Geometry: final body of the model. Coordinates: model frame, mm. Face numbers are marked on the shaded views. A direction names the side the tool comes from. Give positions to 0.01 mm unless a question says otherwise; leave off trailing zeros. Order: outer loops, then holes, each group sorted by start corner. A loop starts at its lowest first (then second) coordinate and runs counter-clockwise, first axis right, second up. Notation, with made-up numbers: M -13,69 L 26,69 A33 cw 26,103 Z; hole C 10.25,-7.5 d10. An arc over 180 degrees is marked long. One line per item, written item: value. Start each with the question number.
```python
from build123d import *

# Parameters (mm, degrees)
SKETCH1_W           = 81.28
SKETCH1_H           = 53.34
BOSS_EXTRUDE1_DEPTH = 22.098
SKETCH2_W           = 27.94
SKETCH2_H           = 22.098
CUT_EXTRUDE1_DEPTH  = 29.591
SKETCH3_W           = 27.94
SKETCH3_H           = 22.098
CUT_EXTRUDE2_DEPTH  = 1.651
SKETCH4_W           = 27.94
SKETCH4_H           = 22.098
CUT_EXTRUDE3_DEPTH  = 29.591
SKETCH5_W           = 27.94
SKETCH5_H           = 22.098
CUT_EXTRUDE4_DEPTH  = 1.651
SKETCH6_W           = 27.94
SKETCH6_H           = 22.098
CUT_EXTRUDE5_DEPTH  = 1.651
CUT_EXTRUDE6_DEPTH  = 8.89
SKETCH8_W           = 27.94
SKETCH8_H           = 22.098
CUT_EXTRUDE7_DEPTH  = 1.651
CUT_EXTRUDE8_DEPTH  = 8.89
SKETCH10_W          = 25.4
SKETCH10_H          = 25.4
BOSS_EXTRUDE2_DEPTH = 1.651
SKETCH11_W          = 25.4
SKETCH11_H          = 25.4
BOSS_EXTRUDE3_DEPTH = 1.651
CUT_EXTRUDE9_DEPTH  = 8.89
CUT_EXTRUDE10_DEPTH = 8.89
CUT_EXTRUDE11_DEPTH = 8.89
CUT_EXTRUDE12_DEPTH = 8.89
CUT_EXTRUDE13_DEPTH = 8.89
CUT_EXTRUDE14_DEPTH = 8.89
CUT_EXTRUDE15_DEPTH = 8.89
CUT_EXTRUDE16_DEPTH = 8.89
CUT_EXTRUDE17_DEPTH = 8.89
CUT_EXTRUDE18_DEPTH = 8.89
SKETCH22_W          = 22.098
SKETCH22_H          = 22.098
BOSS_EXTRUDE4_DEPTH = 27.94
SKETCH23_W          = 15.748
SKETCH23_H          = 15.748
CUT_EXTRUDE19_DEPTH = 27.94
FILLET1_R           = 1.27


with BuildPart() as part:
    # Sketch1 → Boss-Extrude1 (new body)
    with BuildSketch(Plane.XZ.offset(11.049)):
        with Locations((0, 13.97)):
            Rectangle(SKETCH1_W, SKETCH1_H)
    extrude(amount=-BOSS_EXTRUDE1_DEPTH)

    # Sketch2 → Cut-Extrude1 (cut)
    with BuildSketch(Plane.XY.offset(40.64)):
        with Locations((-26.67, 0)):
            Rectangle(SKETCH2_W, SKETCH2_H)
    extrude(amount=-CUT_EXTRUDE1_DEPTH, mode=Mode.SUBTRACT)

    # Sketch3 → Cut-Extrude2 (cut)
    with BuildSketch(Plane(origin=(0, 0, -12.7), x_dir=(-1, 0, 0), z_dir=(0, 0, -1))):
        with Locations((26.67, 0)):
            Rectangle(SKETCH3_W, SKETCH3_H)
    extrude(amount=-CUT_EXTRUDE2_DEPTH, mode=Mode.SUBTRACT)

    # Sketch4 → Cut-Extrude3 (cut)
    with BuildSketch(Plane(origin=(40.64, 0, 0), x_dir=(0, 0, -1), z_dir=(1, 0, 0))):
        with Locations((-26.67, 0)):
            Rectangle(SKETCH4_W, SKETCH4_H)
    extrude(amount=-CUT_EXTRUDE3_DEPTH, mode=Mode.SUBTRACT)

    # Sketch5 → Cut-Extrude4 (cut)
    with BuildSketch(Plane.ZY.offset(12.7)):
        with Locations((26.67, 0)):
            Rectangle(SKETCH5_W, SKETCH5_H)
    extrude(amount=-CUT_EXTRUDE4_DEPTH, mode=Mode.SUBTRACT)

    # Sketch6 → Cut-Extrude5 (cut)
    with BuildSketch(Plane.XY.offset(12.7)):
        with Locations((26.67, 0)):
            Rectangle(SKETCH6_W, SKETCH6_H)
    extrude(amount=-CUT_EXTRUDE5_DEPTH, mode=Mode.SUBTRACT)

    # Sketch7 → Cut-Extrude6 (cut)
    with BuildSketch(Plane(origin=(0, 11.049, 0), x_dir=(-1, 0, 0), z_dir=(0, 1, 0))):
        with BuildLine():
            Line((-12.7, -7.874), (-12.7, 7.874))
            Line((-12.7, 7.874), (-22.1615, 7.874))
            ThreePointArc((-22.1615, 7.874), (-23.1775, 6.858), (-22.1615, 5.842))
            Line((-22.1615, 5.842), (-21.1455, 5.842))
            Line((-21.1455, 5.842), (-21.1455, -5.842))
            Line((-21.1455, -5.842), (-22.1615, -5.842))
            ThreePointArc((-22.1615, -5.842), (-23.1775, -6.858), (-22.1615, -7.874))
            Line((-22.1615, -7.874), (-12.7, -7.874))
        make_face()
    extrude(amount=-CUT_EXTRUDE6_DEPTH, mode=Mode.SUBTRACT)

    # Sketch8 → Cut-Extrude7 (cut)
    with BuildSketch(Plane(origin=(0, 0, -12.7), x_dir=(-1, 0, 0), z_dir=(0, 0, -1))):
        with Locations((-26.67, 0)):
            Rectangle(SKETCH8_W, SKETCH8_H)
    extrude(amount=-CUT_EXTRUDE7_DEPTH, mode=Mode.SUBTRACT)

    # Sketch9 → Cut-Extrude8 (cut)
    with BuildSketch(Plane(origin=(0, 11.049, 0), x_dir=(-1, 0, 0), z_dir=(0, 1, 0))):
        with BuildLine():
            Line((7.874, 12.7), (7.874, 22.1615))
            ThreePointArc((7.874, 22.1615), (6.858, 23.1775), (5.842, 22.1615))
            Line((5.842, 22.1615), (5.842, 21.1455))
            Line((5.842, 21.1455), (-5.842, 21.1455))
            Line((-5.842, 21.1455), (-5.842, 22.1615))
            ThreePointArc((-5.842, 22.1615), (-6.858, 23.1775), (-7.874, 22.1615))
            Line((-7.874, 22.1615), (-7.874, 12.7))
            Line((-7.874, 12.7), (7.874, 12.7))
        make_face()
    extrude(amount=-CUT_EXTRUDE8_DEPTH, mode=Mode.SUBTRACT)

    # Sketch10 → Boss-Extrude2 (add)
    with BuildSketch(Plane(origin=(0, 11.049, 0), x_dir=(-1, 0, 0), z_dir=(0, 1, 0))):
        Rectangle(SKETCH10_W, SKETCH10_H)
    extrude(amount=BOSS_EXTRUDE2_DEPTH)

    # Sketch11 → Boss-Extrude3 (add)
    with BuildSketch(Plane.XZ.offset(11.049)):
        Rectangle(SKETCH11_W, SKETCH11_H)
    extrude(amount=BOSS_EXTRUDE3_DEPTH)

    # Sketch12 → Cut-Extrude9 (cut)
    with BuildSketch(Plane.XZ.offset(11.049)):
        with BuildLine():
            Line((-7.874, 22.1615), (-7.874, 12.7))
            Line((-7.874, 12.7), (7.874, 12.7))
            Line((7.874, 12.7), (7.874, 22.1615))
            ThreePointArc((7.874, 22.1615), (6.858, 23.1775), (5.842, 22.1615))
            Line((5.842, 22.1615), (5.842, 21.1455))
            Line((5.842, 21.1455), (-5.842, 21.1455))
            Line((-5.842, 21.1455), (-5.842, 22.1615))
            ThreePointArc((-5.842, 22.1615), (-6.858, 23.1775), (-7.874, 22.1615))
        make_face()
    extrude(amount=-CUT_EXTRUDE9_DEPTH, mode=Mode.SUBTRACT)

    # Sketch13 → Cut-Extrude10 (cut)
    with BuildSketch(Plane.XZ.offset(11.049)):
        with BuildLine():
            Line((12.7, 7.874), (12.7, -7.874))
            Line((12.7, -7.874), (22.1615, -7.874))
            ThreePointArc((22.1615, -7.874), (23.1775, -6.858), (22.1615, -5.842))
            Line((22.1615, -5.842), (21.1455, -5.842))
            Line((21.1455, -5.842), (21.1455, 5.842))
            Line((21.1455, 5.842), (22.1615, 5.842))
            ThreePointArc((22.1615, 5.842), (23.1775, 6.858), (22.1615, 7.874))
            Line((22.1615, 7.874), (12.7, 7.874))
        make_face()
    extrude(amount=-CUT_EXTRUDE10_DEPTH, mode=Mode.SUBTRACT)

    # Sketch14 → Cut-Extrude11 (cut)
    with BuildSketch(Plane.XZ.offset(11.049)):
        with BuildLine():
            Line((-22.1615, 5.842), (-21.1455, 5.842))
            Line((-21.1455, 5.842), (-21.1455, -5.842))
            Line((-21.1455, -5.842), (-22.1615, -5.842))
            ThreePointArc((-22.1615, -5.842), (-23.1775, -6.858), (-22.1615, -7.874))
            Line((-22.1615, -7.874), (-12.7, -7.874))
            Line((-12.7, -7.874), (-12.7, 7.874))
            Line((-12.7, 7.874), (-22.1615, 7.874))
            ThreePointArc((-22.1615, 7.874), (-23.1775, 6.858), (-22.1615, 5.842))
        make_face()
    extrude(amount=-CUT_EXTRUDE11_DEPTH, mode=Mode.SUBTRACT)

    # Sketch15 → Cut-Extrude12 (cut)
    with BuildSketch(Plane(origin=(0, 11.049, 0), x_dir=(-1, 0, 0), z_dir=(0, 1, 0))):
        with BuildLine():
            Line((21.1455, 5.842), (22.1615, 5.842))
            ThreePointArc((22.1615, 5.842), (23.1775, 6.858), (22.1615, 7.874))
            Line((22.1615, 7.874), (12.7, 7.874))
            Line((12.7, 7.874), (12.7, -7.874))
            Line((12.7, -7.874), (22.1615, -7.874))
            ThreePointArc((22.1615, -7.874), (23.1775, -6.858), (22.1615, -5.842))
            Line((22.1615, -5.842), (21.1455, -5.842))
            Line((21.1455, -5.842), (21.1455, 5.842))
        make_face()
    extrude(amount=-CUT_EXTRUDE12_DEPTH, mode=Mode.SUBTRACT)

    # Sketch16 → Cut-Extrude13 (cut)
    with BuildSketch(Plane.XZ.offset(11.049)):
        with BuildLine():
            Line((-37.465, 7.874), (-37.465, -7.874))
            Line((-37.465, -7.874), (-28.0035, -7.874))
            ThreePointArc((-28.0035, -7.874), (-26.9875, -6.858), (-28.0035, -5.842))
            Line((-28.0035, -5.842), (-29.0195, -5.842))
            Line((-29.0195, -5.842), (-29.0195, 5.842))
            Line((-29.0195, 5.842), (-28.0035, 5.842))
            ThreePointArc((-28.0035, 5.842), (-26.9875, 6.858), (-28.0035, 7.874))
            Line((-28.0035, 7.874), (-37.465, 7.874))
        make_face()
    extrude(amount=-CUT_EXTRUDE13_DEPTH, mode=Mode.SUBTRACT)

    # Sketch17 → Cut-Extrude14 (cut)
    with BuildSketch(Plane.XZ.offset(11.049)):
        with BuildLine():
            Line((28.0035, 5.842), (29.0195, 5.842))
            Line((29.0195, 5.842), (29.0195, -5.842))
            Line((29.0195, -5.842), (28.0035, -5.842))
            ThreePointArc((28.0035, -5.842), (26.9875, -6.858), (28.0035, -7.874))
            Line((28.0035, -7.874), (37.465, -7.874))
            Line((37.465, -7.874), (37.465, 7.874))
            Line((37.465, 7.874), (28.0035, 7.874))
            ThreePointArc((28.0035, 7.874), (26.9875, 6.858), (28.0035, 5.842))
        make_face()
    extrude(amount=-CUT_EXTRUDE14_DEPTH, mode=Mode.SUBTRACT)

    # Sketch18 → Cut-Extrude15 (cut)
    with BuildSketch(Plane(origin=(0, 11.049, 0), x_dir=(-1, 0, 0), z_dir=(0, 1, 0))):
        with BuildLine():
            Line((-29.0195, -5.842), (-29.0195, 5.842))
            Line((-29.0195, 5.842), (-28.0035, 5.842))
            ThreePointArc((-28.0035, 5.842), (-26.9875, 6.858), (-28.0035, 7.874))
            Line((-28.0035, 7.874), (-37.465, 7.874))
            Line((-37.465, 7.874), (-37.465, -7.874))
            Line((-37.465, -7.874), (-28.0035, -7.874))
            ThreePointArc((-28.0035, -7.874), (-26.9875, -6.858), (-28.0035, -5.842))
            Line((-28.0035, -5.842), (-29.0195, -5.842))
        make_face()
    extrude(amount=-CUT_EXTRUDE15_DEPTH, mode=Mode.SUBTRACT)

    # Sketch19 → Cut-Extrude16 (cut)
    with BuildSketch(Plane.XZ.offset(11.049)):
        with BuildLine():
            Line((-7.874, 37.465), (-7.874, 28.0035))
            ThreePointArc((-7.874, 28.0035), (-6.858, 26.9875), (-5.842, 28.0035))
            Line((-5.842, 28.0035), (-5.842, 29.0195))
            Line((-5.842, 29.0195), (5.842, 29.0195))
            Line((5.842, 29.0195), (5.842, 28.0035))
            ThreePointArc((5.842, 28.0035), (6.858, 26.9875), (7.874, 28.0035))
            Line((7.874, 28.0035), (7.874, 37.465))
            Line((7.874, 37.465), (-7.874, 37.465))
        make_face()
    extrude(amount=-CUT_EXTRUDE16_DEPTH, mode=Mode.SUBTRACT)

    # Sketch20 → Cut-Extrude17 (cut)
    with BuildSketch(Plane(origin=(0, 11.049, 0), x_dir=(-1, 0, 0), z_dir=(0, 1, 0))):
        with BuildLine():
            Line((5.842, 29.0195), (5.842, 28.0035))
            ThreePointArc((5.842, 28.0035), (6.858, 26.9875), (7.874, 28.0035))
            Line((7.874, 28.0035), (7.874, 37.465))
            Line((7.874, 37.465), (-7.874, 37.465))
            Line((-7.874, 37.465), (-7.874, 28.0035))
            ThreePointArc((-7.874, 28.0035), (-6.858, 26.9875), (-5.842, 28.0035))
            Line((-5.842, 28.0035), (-5.842, 29.0195))
            Line((-5.842, 29.0195), (5.842, 29.0195))
        make_face()
    extrude(amount=-CUT_EXTRUDE17_DEPTH, mode=Mode.SUBTRACT)

    # Sketch21 → Cut-Extrude18 (cut)
    with BuildSketch(Plane(origin=(0, 11.049, 0), x_dir=(-1, 0, 0), z_dir=(0, 1, 0))):
        with BuildLine():
            Line((28.0035, -7.874), (37.465, -7.874))
            Line((37.465, -7.874), (37.465, 7.874))
            Line((37.465, 7.874), (28.0035, 7.874))
            ThreePointArc((28.0035, 7.874), (26.9875, 6.858), (28.0035, 5.842))
            Line((28.0035, 5.842), (29.0195, 5.842))
            Line((29.0195, 5.842), (29.0195, -5.842))
            Line((29.0195, -5.842), (28.0035, -5.842))
            ThreePointArc((28.0035, -5.842), (26.9875, -6.858), (28.0035, -7.874))
        make_face()
    extrude(amount=-CUT_EXTRUDE18_DEPTH, mode=Mode.SUBTRACT)

    # Sketch22 → Boss-Extrude4 (add)
    with BuildSketch(Plane(origin=(0, 12.7, 0), x_dir=(-1, 0, 0), z_dir=(0, 1, 0))):
        Rectangle(SKETCH22_W, SKETCH22_H)
    extrude(amount=BOSS_EXTRUDE4_DEPTH)

    # Sketch23 → Cut-Extrude19 (cut)
    with BuildSketch(Plane(origin=(0, 40.64, 0), x_dir=(-1, 0, 0), z_dir=(0, 1, 0))):
        Rectangle(SKETCH23_W, SKETCH23_H)
    extrude(amount=-CUT_EXTRUDE19_DEPTH, mode=Mode.SUBTRACT)

    # Fillet1
    fillet1_edges = [part.edges().sort_by_distance(p)[0] for p in [
        (26.67, 11.049, -11.049),
        (26.67, -11.049, -11.049),
        (-26.67, 11.049, 11.049),
        (-26.67, -11.049, 11.049),
        (-26.67, -11.049, -11.049),
        (-26.67, 11.049, -11.049),
        (-11.049, 26.67, -11.049),
        (-11.049, 26.67, 11.049),
        (11.049, 26.67, 11.049),
        (11.049, 26.67, -11.049),
        (11.049, -11.049, 26.67),
        (11.049, 11.049, 26.67),
        (-11.049, 11.049, 26.67),
        (-11.049, -11.049, 26.67),
        (26.67, -11.049, 11.049),
        (26.67, 11.049, 11.049),
    ]]
    fillet(fillet1_edges, radius=FILLET1_R)


solid = part.part
```
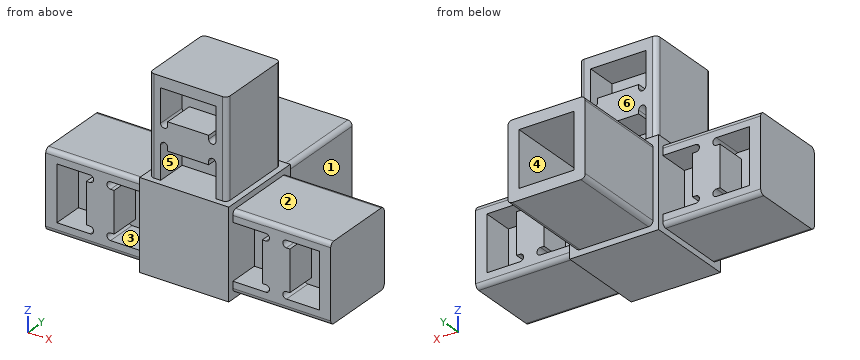
Q1. Set-up query: the marked faces 4, 5 and 6. Return all of +Z, -Z, +X, -X, +Y, -Y with unobstructed straight access to the full face (end or side cutting, diameter ignored); none if empty.
Q2. Mould query, pull axis Z, two halves, no side actions, for the marked faces 1, 2 and 3. Classes: +Z half, -Z half, draft (parallel to the pull), parting line (faces both ways), or undercut.
Q3. Section query D-D on x = 32. Return loops of the section in (y, z), and give its area (3 significant figures).
Q4. Section query C-C on z = 32.5. Return loops of the section in (x, y).
Q5. Ray query, line 1 along X through (y, z) = (9, 2) (1 decimal); line 2 along Z through (x, y) = (-1.5, -9.5) (1 decimal); line 3 along X through (y, z) = (26, -2.5). Return the intervals inside material, ascending. Write a range as [from, to].
Q6. Section query A-A on y = 25.5. Return loops of the section in (x, z), and give its area (3 significant figures).
Q7. Section query B-B on x = 1. Return loops of the section in (y, z) (1 decimal).
Q8. Contact query for flat-ended pins moving along their axis: pin 1 (2 mm diameter, centred on x = -8.5, y = 14.5, fed in from -Z); pin 2 (15.5 mm diameter, centred on y = -3, z = 20.5, fed in from -X); pin 3 (8 mm diameter, centred on x = -1.5, y = 21.5, fed in from +Z). Output: stop coordinate, or through.
Results below:
1. face 4: +Y
1. face 5: -Y
1. face 6: +Z, +X, -X, +Y
2. face 1: draft
2. face 2: +Z half
2. face 3: undercut
3. outline: M -11.05,-9.78 A1.27 ccw -9.78,-11.05 L 9.78,-11.05 A1.27 ccw 11.05,-9.78 L 11.05,-7.87 L 2.16,-7.87 L 2.16,7.87 L 11.05,7.87 L 11.05,9.78 A1.27 ccw 9.78,11.05 L -9.78,11.05 A1.27 ccw -11.05,9.78 L -11.05,7.87 L -2.16,7.87 L -2.16,-7.87 L -11.05,-7.87 Z
3. area: 207 mm2
4. outline: M -11.05,-9.78 A1.27 ccw -9.78,-11.05 L -7.87,-11.05 L -7.87,-2.16 L 7.87,-2.16 L 7.87,-11.05 L 9.78,-11.05 A1.27 ccw 11.05,-9.78 L 11.05,9.78 A1.27 ccw 9.78,11.05 L 7.87,11.05 L 7.87,2.16 L -7.87,2.16 L -7.87,11.05 L -9.78,11.05 A1.27 ccw -11.05,9.78 Z
5. line 1: [-40.6, -37.5], [-29, -21.1], [-12.7, 12.7], [21.1, 29], [37.5, 40.6]
5. line 2: [-12.7, 12.7], [21.1, 29], [37.5, 40.6]
5. line 3: [-11.05, -7.87], [7.87, 11.05]
6. outline: M -11.05,-9.78 A1.27 ccw -9.78,-11.05 L 9.78,-11.05 A1.27 ccw 11.05,-9.78 L 11.05,9.78 A1.27 ccw 9.78,11.05 L -9.78,11.05 A1.27 ccw -11.05,9.78 Z; hole M -7.87,-7.87 L 7.87,-7.87 L 7.87,7.87 L -7.87,7.87 Z
6. area: 239 mm2
7. outline: M -12.7,-12.7 L 12.7,-12.7 L 12.7,-11 L 40.6,-11 L 40.6,-7.9 L 12.7,-7.9 L 12.7,7.9 L 40.6,7.9 L 40.6,11 L 12.7,11 L 12.7,12.7 L 2.2,12.7 L 2.2,21.1 L 11,21.1 L 11,29 L 2.2,29 L 2.2,37.5 L 11,37.5 L 11,40.6 L -11,40.6 L -11,37.5 L -2.2,37.5 L -2.2,29 L -11,29 L -11,21.1 L -2.2,21.1 L -2.2,12.7 L -12.7,12.7 Z
8. pin 1: z = -11.05
8. pin 2: x = -11.05
8. pin 3: z = 11.05
